Input: part model. Units: mm. Frame: model coordinates. Give positions to 0.01 mm unless a question says otherwise; leave off trailing zeros. Write each loop counter-clockwise with the first axis right and the second up, starting at its lowest first coordinate (ties: lowest second). Pieces come first, ordered by that corner, then holes. Notation, with made-up numbers: (41, 39.5) - (46, 39.5) arc R22 cw to (46, 66.5) - close; hole circle Ø11 at (40.25, 59). An arc over 180 degrees is marked (long way). Answer as CSV lines item,"result".
Autodesk Inventor part; units mm, degrees
ref_plane "YZ Plane" through (0, 0, 0) normal (1, 0, 0) x (0, 1, 0)
ref_plane "XZ Plane" through (0, 0, 0) normal (0, 1, 0) x (-1, 0, 0)
ref_plane "XY Plane" through (0, 0, 0) normal (0, 0, 1) x (1, 0, 0)
sketch "Boceto1" plane through (0, 0, 0) normal (0, 0, 1) x (1, 0, 0)
  line L0 (0, 0) -> (75, 0)
  line L1 (75, 0) -> (75, 12.7)
  line L2 (75, 12.7) -> (0, 12.7)
  line L3 (0, 12.7) -> (0, 0)
  dimension "d0" = 75
  dimension "d1" = 12.7
extrude "Extrusión1" add sketch "Boceto1" along normal blind 12.7
sketch "Boceto2" plane through (0, 0, 0) normal (0, 0, -1) x (-1, 0, 0)
  line L0 (0, 12.7) -> (0, 0)
  line L1 (0, 6.35) -> (-28.6, 6.35)
  line L2 (-28.6, 6.35) -> (-34.05, 6.35)
  line L3 (-28.6, 6.35) -> (-23.15, 6.35) construction
  circle A0 centre (-34.05, 6.35) radius 5.45
  line L4 (-75, 6.35) -> (-46.4, 6.35)
  line L5 (-46.4, 6.35) -> (-40.95, 6.35)
  line L6 (-46.4, 6.35) -> (-51.85, 6.35) construction
  circle A1 centre (-40.95, 6.35) radius 5.45
  point P0 (-37.5, 2.131)
  point P1 (-37.5, 10.569)
  dimension "d4" = 28.6
  dimension "d5" = 5.45
  dimension "d6" = 180
  dimension "d7" = 28.6
  dimension "d8" = 5.45
  dimension "d9" = 180
extrude "Extrusión2" cut sketch "Boceto2" against normal blind 12.7
sketch "Boceto3" plane through (0, 0, 0) normal (0, -1, 0) x (1, 0, 0)
  line L0 (75, 0) -> (75, 12.7)
  line L1 (75, 6.35) -> (71.1, 6.35)
  line L2 (71.1, 6.35) -> (69.375, 6.35)
  circle A0 centre (69.375, 6.35) radius 1.725
  line L3 (67.65, 6.35) -> (60.9, 6.35)
  line L4 (60.9, 6.35) -> (59.175, 6.35)
  circle A1 centre (59.175, 6.35) radius 1.725
  circle A2 centre (69.375, 6.35) radius 2
  circle A3 centre (59.175, 6.35) radius 2
  line L5 (75, 0) -> (0, 0)
  line L6 (37.5, 0) -> (37.5, 12.7)
  line L7 (0, 12.7) -> (75, 12.7)
  line L8 (0, 6.4) -> (3.9, 6.4)
  line L9 (3.9, 6.4) -> (5.625, 6.4)
  circle A4 centre (5.625, 6.4) radius 1.725
  line L10 (7.35, 6.4) -> (14.1, 6.4)
  line L11 (14.1, 6.4) -> (15.825, 6.4)
  circle A5 centre (15.825, 6.4) radius 1.725
  circle A6 centre (5.625, 6.4) radius 2
  circle A7 centre (15.825, 6.4) radius 2
  line L12 (0, 0) -> (75, 0)
  dimension "d12" = 3.9
  dimension "d13" = 1.725
  dimension "d14" = 6.75
  dimension "d15" = 1.725
  dimension "d16" = 4
  dimension "d17" = 4
  dimension "d18" = 3.9
  dimension "d19" = 1.725
  dimension "d20" = 6.75
  dimension "d21" = 1.725
  dimension "d22" = 4
  dimension "d23" = 4
  dimension "d31" = 6.4
  dimension "d32" = 6.4
hole "Agujero1" at (59.175, 0, 6.35) at (69.375, 0, 6.35) at (15.825, 0, 6.4) at (5.625, 0, 6.4) direction (0, 1, 0) diameter 4 depth 12.7
properties part number "Celda_Carga"
Item 1: Mould query, pull axis Y, two halves, no side actions, for faces 1 (the face through (67.39, 6.44, 6.61)), 2 (the face through (28.603, 6.178, 6.261)), 3 (the face through (37, 0, 6)). Classes: +Y half, -Y half, draft (parallel to the pull), parting line (faces both ways), or undercut.
The answers:
face 1,"draft"
face 2,"undercut"
face 3,"-Y half"
Item 2: Cut plane A-A on x = 40.95. Return the cut outline in (y, z).
The answers:
outline,"(0, 0) - (0.9, 0) - (0.9, 12.7) - (0, 12.7) - close; (11.8, 0) - (12.7, 0) - (12.7, 12.7) - (11.8, 12.7) - close"
Item 3: Cut plane B-B on z = 6.35. Return the cut outline in (x, y) (3 decimals).
The answers:
outline,"(0, 0) - (3.626, 0) - (3.626, 12.7) - (0, 12.7) - close; (7.624, 0) - (13.826, 0) - (13.826, 12.7) - (7.624, 12.7) - close; (17.824, 0) - (57.175, 0) - (57.175, 12.7) - (17.824, 12.7) - close; (61.175, 0) - (67.375, 0) - (67.375, 12.7) - (61.175, 12.7) - close; (71.375, 0) - (75, 0) - (75, 12.7) - (71.375, 12.7) - close; hole (37.5, 2.131) arc R5.45 ccw (long way) to (37.5, 10.569) arc R5.45 ccw (long way) to start"
Item 4: Cut plane C-C on y = 6.35. Return the cut outline in (x, z) (3 decimals), plus the area to 3 significant figures.
The answers:
outline,"(0, 0) - (28.6, 0) - (28.6, 12.7) - (0, 12.7) - close; (46.4, 0) - (75, 0) - (75, 12.7) - (46.4, 12.7) - close; hole circle Ø4 at (5.625, 6.4); hole circle Ø4 at (15.825, 6.4); hole circle Ø4 at (59.175, 6.35); hole circle Ø4 at (69.375, 6.35)"
area,"676 mm²"
Item 5: Ray query, line 1 (X direction, y = 6, z = 6.4) (3 decimals); line 2 (Y direction, x = 40.95, z = 8.25); line 3 (Z direction, x = 5.5, y = 10.5). Return the intervals inside material, ascending. Write a range as from..to.
The answers:
line 1,"0..3.625, 7.625..13.825, 17.825..28.611, 46.389..57.176, 61.174..67.376, 71.374..75"
line 2,"0..0.9, 11.8..12.7"
line 3,"0..4.4, 8.4..12.7"
Item 6: Cut plane D-D on z = 3.5. Return the cut outline in (x, y).
The answers:
outline,"(0, 0) - (75, 0) - (75, 12.7) - (0, 12.7) - close; hole (37.5, 2.13) arc R5.45 ccw (long way) to (37.5, 10.57) arc R5.45 ccw (long way) to start"
